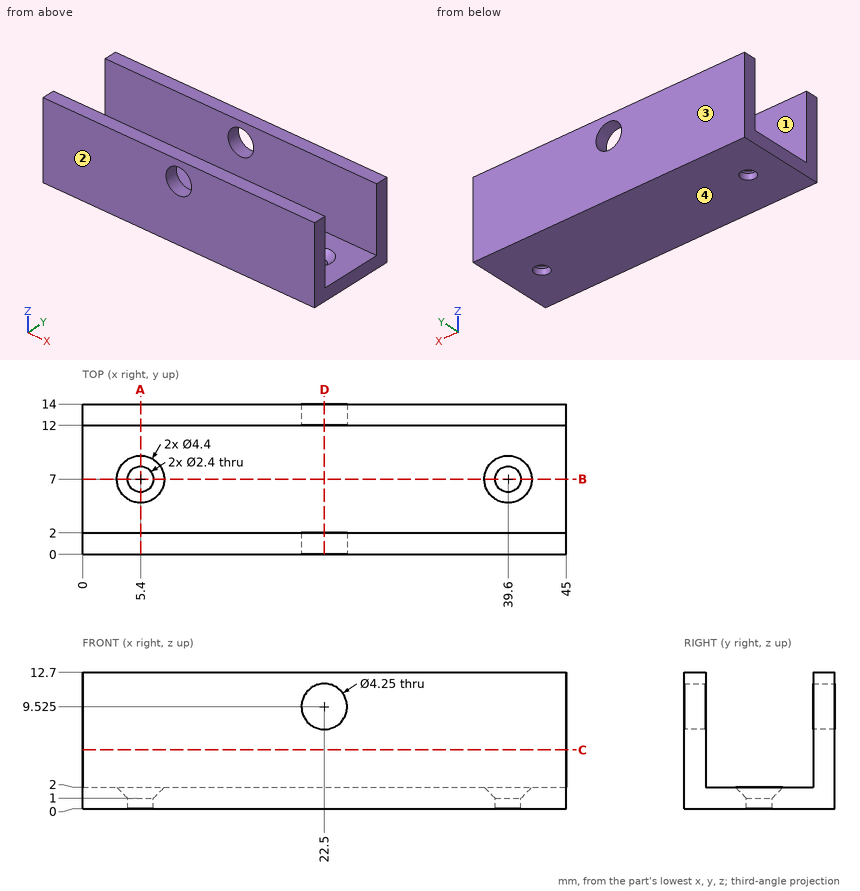
Geometry: see drawing. Coordinates: mm, zero at the bounding-box minimum. Round coordinates to 2 decimals unless told otherwise and drop trailing zeros. Write each loop counter-clockwise with the first axis right and the second up, starting at its lowest first coordinate (ties: lowest second). Pieces come first, ordered by that corner, then holes.
1) Cut plane D-D (x = 22.5). Return the cut outline in (y, z).
2) Cut plane B-B (y = 7). Return the cut outline in (x, z), then the cut area to 3 significant figures.
3) Draft query along Y for the marked faces 1, 2, 3 and 4. Return one class per face: pulls with the +Y half, pulls with the -Y half, needs draft (parallel to the pull), parting line crosses it, or undercut.
4) Cut plane C-C (z = 5.5). Return the cut outline in (x, y), then the cut area to 3 significant figures.
5) Cut plane A-A (x = 5.4). Return the cut outline in (y, z).
6) Contact query for flat-ended pins moving along their axis: P1, Ø5.5, axis at x = 22.5, z = 9.525, coming from the +Y side; P2, Ø1.5, axis at x = 14, y = 5.5, coming from the +Z side; P3, Ø4, axis at x = 5.4, y = 7, coming from the +Z side. Output: stop coordinate, or through.
7) Ray query, L1, parallel to X at y = 7, z = 0.3; L2, parallel to Z at x = 22.5, y = 0.75; L3, parallel to Y at x = 39.6, z = 0.65. Return the intervals inside material, ascending.
Geometry says:
1. outline: (0, 0) - (14, 0) - (14, 7.4) - (12, 7.4) - (12, 2) - (2, 2) - (2, 7.4) - (0, 7.4) - close; (0, 11.65) - (2, 11.65) - (2, 12.7) - (0, 12.7) - close; (12, 11.65) - (14, 11.65) - (14, 12.7) - (12, 12.7) - close
2. outline: (0, 0) - (4.2, 0) - (4.2, 1) - (3.2, 2) - (0, 2) - close; (6.6, 0) - (38.4, 0) - (38.4, 1) - (37.4, 2) - (7.6, 2) - (6.6, 1) - close; (40.8, 0) - (45, 0) - (45, 2) - (41.8, 2) - (40.8, 1) - close
2. area: 78.4 mm2
3. face 1: undercut
3. face 2: pulls with the -Y half
3. face 3: pulls with the +Y half
3. face 4: needs draft
4. outline: (0, 0) - (45, 0) - (45, 2) - (0, 2) - close; (0, 12) - (45, 12) - (45, 14) - (0, 14) - close
4. area: 180 mm2
5. outline: (0, 0) - (5.8, 0) - (5.8, 1) - (4.8, 2) - (2, 2) - (2, 12.7) - (0, 12.7) - close; (8.2, 0) - (14, 0) - (14, 12.7) - (12, 12.7) - (12, 2) - (9.2, 2) - (8.2, 1) - close
6. P1: stops at y = 14
6. P2: stops at z = 2
6. P3: stops at z = 1.8
7. L1: x = 0 to 4.2, 6.6 to 38.4, 40.8 to 45
7. L2: z = 0 to 7.4, 11.65 to 12.7
7. L3: y = 0 to 5.8, 8.2 to 14
